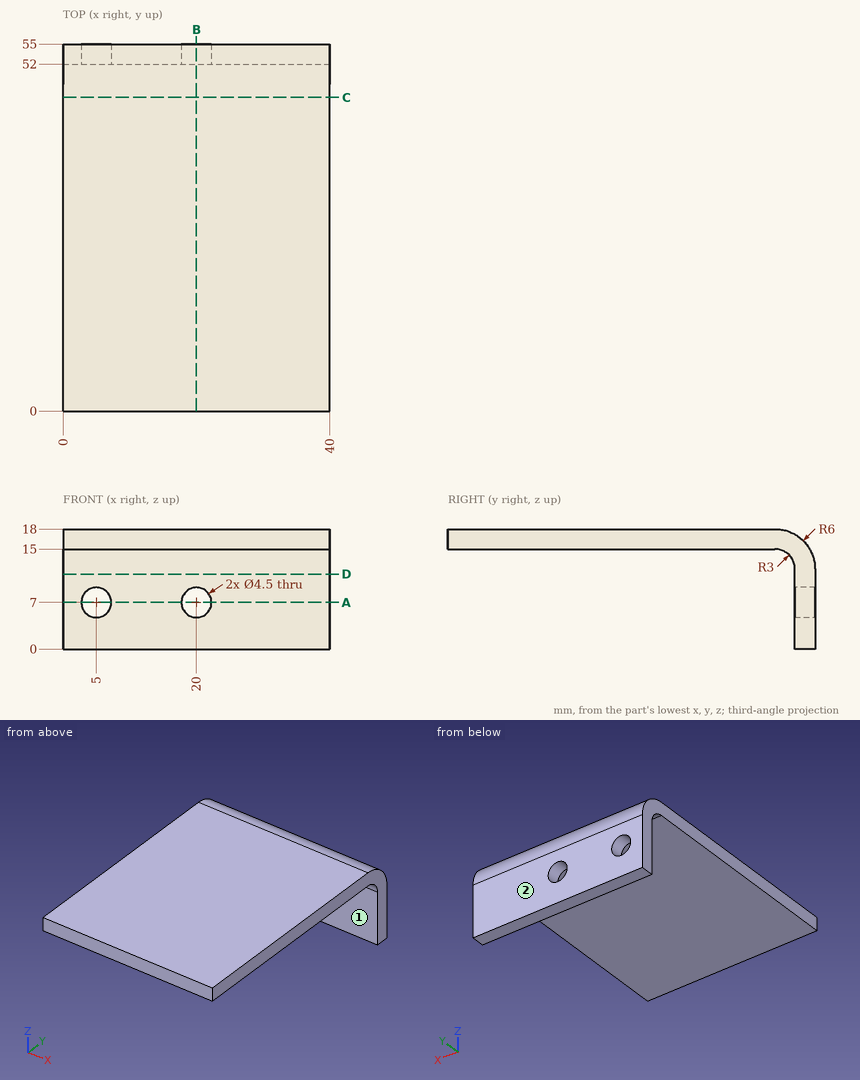
Study the drawing (mm; zero at the part's minimum x, y, z) and answer. A direction names the side the tool comes from. Coordinates: 2 decimals unless noted, no trailing zeros. Write each loop counter-clockwise with the first axis right and the second up, starting at its lowest first coordinate (ties: lowest second). Pieces come first, ordered by that corner, then holes. Notation, with made-up numbers: (-35, 27) - (1, 27) arc R18 ccw to (1, 45) - close; hole circle Ø4 at (47, 77). An arc over 180 degrees is marked (long way). Return JSON: item names as keys, results as strings. Group by question number.
1. Which of the six approach directions +Z, -Z, +X, -X, +Y, -Y give full straight-line access (tool end or side, diameter ignored) to the marked faces 1 and 2?
2. A cutting plane is placed at A-A, the plane z = 7. Determine the outline of the cut face in (x, y), plus the area to 3 significant figures.
3. Straight lines are drawn through the part: L1, parallel to X at y = 53.9, z = 7; L2, parallel to Y at x = 4, z = 3.75; L3, parallel to Z at x = 4, y = 9. For each, find the intervals that lie inside material, in ascending order.
4. Given pin 1 (2 mm diameter, centred on x = 32, y = 7, fed in from -Z); pin 2 (10 mm diameter, centred on x = 14, z = 5.5, fed in from -Y); pin 3 (6 mm diameter, centred on x = 28.5, z = 10, fed in from -Y), each flat-ended and moving along its own axis, determine where each tip first touches the part or whether it passes through.
5. A cutting plane is placed at C-C, the plane y = 47. Determine the outline of the cut face in (x, z).
6. A cutting plane is placed at B-B, the plane x = 20. Determine the outline of the cut face in (y, z), plus the area to 3 significant figures.
7. A cutting plane is placed at D-D, the plane z = 11.25. Determine the outline of the cut face in (x, y), plus the area to 3 significant figures.
Ans:
{
 "1": {"face 1": "-Z, +X, -X, -Y", "face 2": "+Z, -Z, +X, -X, +Y"},
 "2": {"outline": "(0, 52) - (2.75, 52) - (2.75, 55) - (0, 55) - close; (7.25, 52) - (17.75, 52) - (17.75, 55) - (7.25, 55) - close; (22.25, 52) - (40, 52) - (40, 55) - (22.25, 55) - close", "area": "93.0 mm²"},
 "3": {"L1": "0 to 2.75, 7.25 to 17.75, 22.25 to 40", "L2": "52 to 55", "L3": "15 to 18"},
 "4": {"pin 1": "z = 15", "pin 2": "y = 52", "pin 3": "y = 51.83"},
 "5": {"outline": "(0, 15) - (40, 15) - (40, 18) - (0, 18) - close"},
 "6": {"outline": "(0, 15) - (49, 15) arc R3 cw to (52, 12) - (52, 9.25) - (55, 9.25) - (55, 12) arc R6 ccw to (49, 18) - (0, 18) - close; (52, 0) - (55, 0) - (55, 4.75) - (52, 4.75) - close", "area": "191 mm²"},
 "7": {"outline": "(0, 52) - (40, 52) - (40, 55) - (0, 55) - close", "area": "120 mm²"}
}
